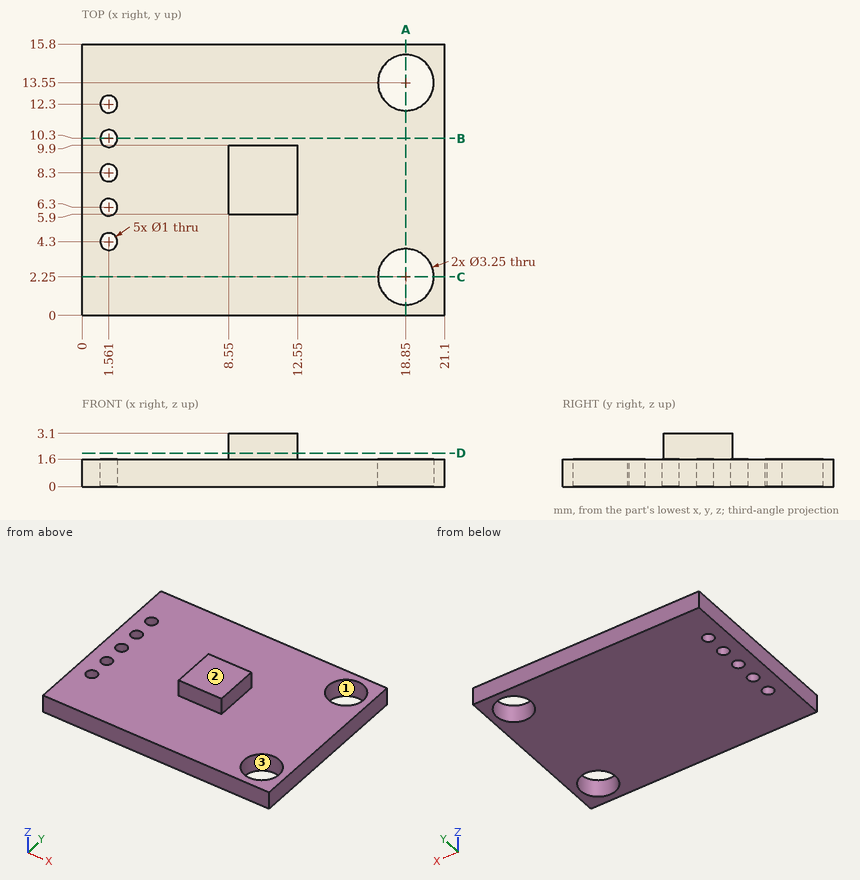
For this review, use the dimensioned drawing (mm, ordinates from the lowest corner) and the shaded views. Round coordinates to 2 decimals unless told otherwise and drop trailing zeros. Write each loop counter-clockwise with the first axis right and the second up, starting at its lowest first coordinate (ties: lowest second). Pieces come first, ordered by that corner, then holes. Notation, with made-up numbers: (72, 17) - (115, 17) arc R7 ccw to (115, 30) - close; hole circle Ø5 at (-39.75, 7). An arc over 180 degrees is marked (long way). Answer as a JSON object with one key per item and string values.
1. We need section C-C on y = 2.25. Give the boundary of the cut face in (x, z) (1 decimal).
Response values:
{"outline": "(0, 0) - (17.2, 0) - (17.2, 1.6) - (0, 1.6) - close; (20.5, 0) - (21.1, 0) - (21.1, 1.6) - (20.5, 1.6) - close"}
2. We need section B-B on y = 10.3. Give the boundary of the cut face in (x, z).
Response values:
{"outline": "(0, 0) - (1.06, 0) - (1.06, 1.6) - (0, 1.6) - close; (2.06, 0) - (21.1, 0) - (21.1, 1.6) - (2.06, 1.6) - close"}
3. We need section A-A on x = 18.85. Give the boundary of the cut face in (y, z) (1 decimal).
Response values:
{"outline": "(0, 0) - (0.6, 0) - (0.6, 1.6) - (0, 1.6) - close; (3.9, 0) - (11.9, 0) - (11.9, 1.6) - (3.9, 1.6) - close; (15.2, 0) - (15.8, 0) - (15.8, 1.6) - (15.2, 1.6) - close"}
4. We need section D-D on z = 1.95. Give the boundary of the cut face in (x, y), then the cut area to 3 significant figures.
Response values:
{"outline": "(8.55, 5.9) - (12.55, 5.9) - (12.55, 9.9) - (8.55, 9.9) - close", "area": "16.0 mm2"}
5. To check wall thickness, follow line 1 along Y through (x, z) = (18.85, 1.2) (1 decimal); line 2 along Y through (x, z) = (1.5, 0.25); line 3 along X through (y, z) = (12.5, 1). State the ranges of each line that lie inside material, in increasing order.
Response values:
{"line 1": "y = 0 to 0.6, 3.9 to 11.9, 15.2 to 15.8", "line 2": "y = 0 to 3.8, 4.8 to 5.8, 6.8 to 7.8, 8.8 to 9.8, 10.8 to 11.8, 12.8 to 15.8", "line 3": "x = 0 to 1.1, 2.02 to 17.61, 20.09 to 21.1"}
6. Draft analysis for pull direction Y (two halves, no side actions). For the marked faces 1, 2 and 3, state which applies: +Y half, -Y half, draft (parallel to the pull), parting line (faces both ways), or undercut.
Response values:
{"face 1": "undercut", "face 2": "draft", "face 3": "undercut"}
7. For pin 1 Ø1.5 at (x, y) = (3.5, 6) entering from +Z; pin 2 Ø3 at (x, y) = (18.85, 13.55) entering from -Z; pin 3 Ø1.6 at (x, z) = (10.5, 2.5) entering from +Y, all flat-tipped, find the tip position at first contact; note any pin that passes through.
Response values:
{"pin 1": "stops at z = 1.6", "pin 2": "passes through", "pin 3": "stops at y = 9.9"}
